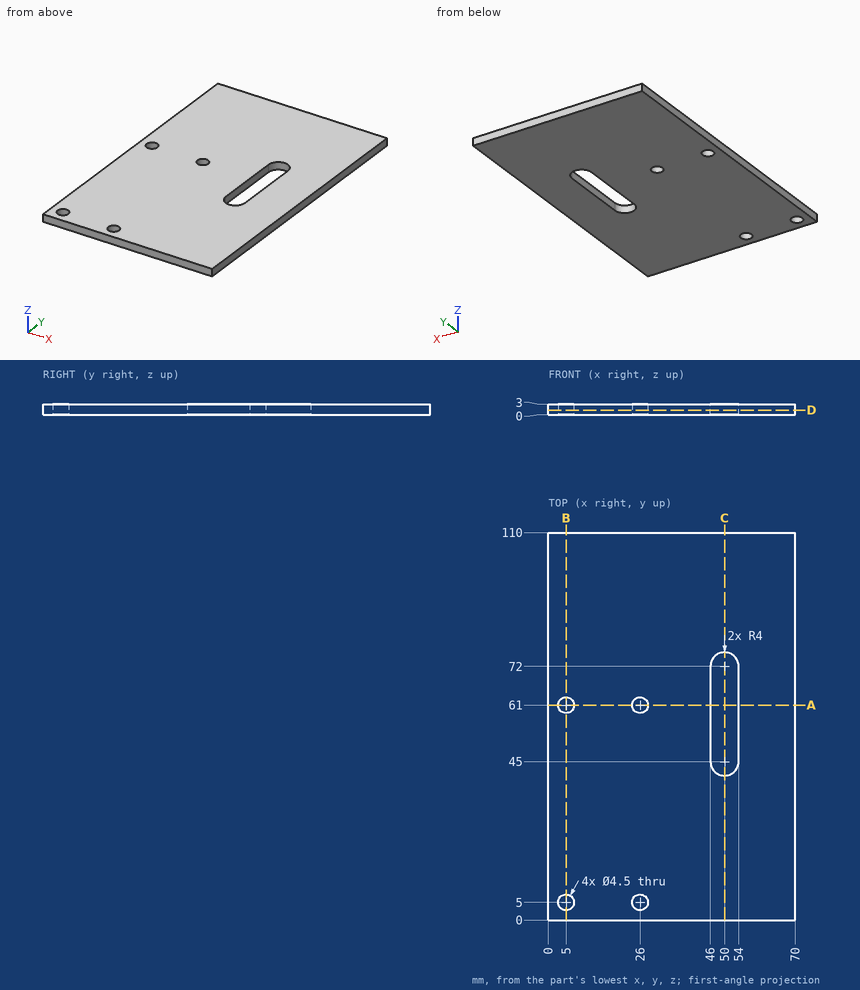
Drawing for the job (mm, zero at the part's lowest x, y, z). Round coordinates to 2 decimals unless told otherwise and drop trailing zeros. Write each loop counter-clockwise with the first axis right and the second up, starting at its lowest first coordinate (ties: lowest second). Pieces come first, ordered by that corner, then holes. Notation, with made-up numbers: M 45.5,71 L 90.5,71 A18 cw 90.5,87 Z; hole C -3,24 d10. An arc over 180 degrees is marked long. One line per question, with ' | ' between items.
1. Cut at B-B on x = 5. Write the cut outline in (y, z).
Working result:
outline: M 0,0 L 2.75,0 L 2.75,3 L 0,3 Z; M 7.25,0 L 58.75,0 L 58.75,3 L 7.25,3 Z; M 63.25,0 L 110,0 L 110,3 L 63.25,3 Z
2. Probe L1, parallel to Y at x = 26, z = 2.1; L2, parallel to X at y = 55.5, z = 1.3; L3, parallel to Y at x = 24, z = 1.45. List the from-to ranges inside material, lowest first. Write a range as from..to.
Working result:
L1: 0..2.75, 7.25..58.75, 63.25..110 | L2: 0..46, 54..70 | L3: 0..3.97, 6.03..59.97, 62.03..110
3. Cut at C-C on x = 50. Write the cut outline in (y, z), and give its area (3 significant figures).
Working result:
outline: M 0,0 L 41,0 L 41,3 L 0,3 Z; M 76,0 L 110,0 L 110,3 L 76,3 Z | area: 225 mm2
4. Cut at D-D on z = 1.25. Write the cut outline in (x, y).
Working result:
outline: M 0,0 L 70,0 L 70,110 L 0,110 Z; hole C 5,5 d4.5; hole C 5,61 d4.5; hole C 26,5 d4.5; hole C 26,61 d4.5; hole M 46,45 A4 ccw 54,45 L 54,72 A4 ccw 46,72 Z
5. Cut at A-A on y = 61. Write the cut outline in (x, z), and give its area (3 significant figures).
Working result:
outline: M 0,0 L 2.75,0 L 2.75,3 L 0,3 Z; M 7.25,0 L 23.75,0 L 23.75,3 L 7.25,3 Z; M 28.25,0 L 46,0 L 46,3 L 28.25,3 Z; M 54,0 L 70,0 L 70,3 L 54,3 Z | area: 159 mm2
